```python
from build123d import *

# Parameters (mm, degrees)
SKETCH1_W           = 15
SKETCH1_H           = 70
BOSS_EXTRUDE1_DEPTH = 3


with BuildPart() as part:
    # Sketch1 → Boss-Extrude1 (new body)
    with BuildSketch(Plane(origin=(0, 0, 0), x_dir=(1, 0, 0), z_dir=(0, 1, 0))):
        with Locations((7.5, 35)):
            Rectangle(SKETCH1_W, SKETCH1_H)
        Polygon((9.08771324, 7.75), (5.91228676, 7.75), (4.324573519, 5), (5.91228676, 2.25), (9.08771324, 2.25), (10.675426481, 5), align=None, mode=Mode.SUBTRACT)
        Polygon((9.08771324, 62.25), (5.91228676, 62.25), (4.324573519, 65), (5.91228676, 67.75), (9.08771324, 67.75), (10.675426481, 65), align=None, mode=Mode.SUBTRACT)
    extrude(amount=BOSS_EXTRUDE1_DEPTH)


solid = part.part
```
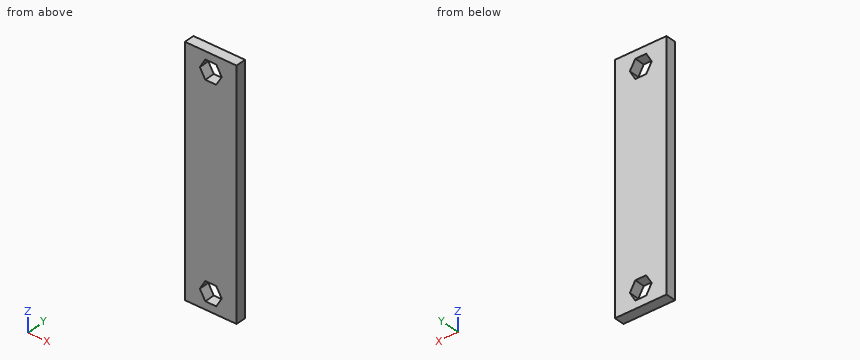
Here's how the part is built. I have some questions about the finished solid (model axes, mm). Coordinates: 2 decimals unless noted, no trailing zeros. Order: outer loops, then holes, each group sorted by start corner. A loop starts at its lowest first (then second) coordinate and runs counter-clockwise, first axis right, second up. Notation, with made-up numbers: M 33.5,-23.75 L 81.5,-23.75 A32 cw 81.5,13.25 Z; hole C -6,-18 d3. An arc over 180 degrees is marked long. Answer as a JSON object with one key per item and string values. Group by question number.
(1) I need wall thicknesses on probe 1 along Z at (x, y) = (6.25, 2.5); probe 2 along Z at (x, y) = (5.25, 1.2); probe 3 along X at (y, z) = (2.8, -65). Which ranges of each line are inside material? Lowest first, please.
(2) Suppose I cut it at A-A, the plane x = 6.75. Please give me the cut outline in (y, z).
(3) Suppose I cut it at B-B, the plane y = 1.3. Please give me the cut outline in (x, z).
Values found:
{
 "1": {"probe 1": "z = -70 to -67.75, -62.25 to -7.75, -2.25 to 0", "probe 2": "z = -70 to -66.6, -63.4 to -6.6, -3.4 to 0", "probe 3": "x = 0 to 4.32, 10.68 to 15"},
 "2": {"outline": "M 0,-70 L 3,-70 L 3,-67.75 L 0,-67.75 Z; M 0,-62.25 L 3,-62.25 L 3,-7.75 L 0,-7.75 Z; M 0,-2.25 L 3,-2.25 L 3,0 L 0,0 Z"},
 "3": {"outline": "M 0,-70 L 15,-70 L 15,0 L 0,0 Z; hole M 4.32,-65 L 5.91,-67.75 L 9.09,-67.75 L 10.68,-65 L 9.09,-62.25 L 5.91,-62.25 Z; hole M 4.32,-5 L 5.91,-7.75 L 9.09,-7.75 L 10.68,-5 L 9.09,-2.25 L 5.91,-2.25 Z"}
}
